from build123d import *

# Parameters (mm, degrees)
CROQUIS5_R              = 1.6
SALIENTE_EXTRUIR3_DEPTH = 15
SALIENTE_EXTRUIR5_DEPTH = 2
CORTAR_EXTRUIR3_DEPTH   = 3
CROQUIS10_W             = 4
CROQUIS10_H             = 50
SALIENTE_EXTRUIR6_DEPTH = 18
CROQUIS17_R             = 1.6
CORTAR_EXTRUIR4_DEPTH   = 4
CORTAR_EXTRUIR6_DEPTH   = 3


with BuildPart() as part:
    # Croquis5 → Saliente-Extruir3 (new body)
    with BuildSketch(Plane(origin=(0, 0, 0), x_dir=(1, 0, 0), z_dir=(0, 1, 0))):
        with BuildLine():
            Line((-65.609813571, 16.762782914), (-61.088751749, 16.762782914))
            ThreePointArc((-61.088751749, 16.762782914), (-59.34928266, 13.462782914), (-61.088751749, 10.162782914))
            Line((-61.088751749, 10.162782914), (-65.609813571, 10.162782914))
            ThreePointArc((-65.609813571, 10.162782914), (-67.34928266, 13.462782914), (-65.609813571, 16.762782914))
        make_face()
        with Locations(Location((-63.34928266, 13.462782914, 0), (0, 0, 270))):
            Circle(CROQUIS5_R, mode=Mode.SUBTRACT)
    extrude(amount=SALIENTE_EXTRUIR3_DEPTH)

    # Croquis7 → Saliente-Extruir5 (add)
    with BuildSketch(Plane(origin=(0, 15, 0), x_dir=(1, 0, 0), z_dir=(0, 1, 0))):
        Polygon((-63.34928266, 13.462782914), (-63.34928266, -11.537217086), (-71.34928266, -11.537217086), (-71.34928266, 38.462782914), (-63.34928266, 38.462782914), align=None)
    extrude(amount=-SALIENTE_EXTRUIR5_DEPTH)

    # Croquis9 → Cortar-Extruir3 (cut)
    with BuildSketch(Plane(origin=(0, 15, 0), x_dir=(1, 0, 0), z_dir=(0, 1, 0))):
        Polygon((-60.274222832, 14.551286652), (-62.754424635, 16.670114712), (-65.829484463, 15.581610975), (-66.424342488, 12.374279177), (-63.944140685, 10.255451116), (-60.869080857, 11.343954853), align=None)
    extrude(amount=-CORTAR_EXTRUIR3_DEPTH, mode=Mode.SUBTRACT)

    # Croquis10 → Saliente-Extruir6 (add)
    with BuildSketch(Plane(origin=(0, 15, 0), x_dir=(1, 0, 0), z_dir=(0, 1, 0))):
        with Locations((-69.34928266, 13.462782914)):
            Rectangle(CROQUIS10_W, CROQUIS10_H)
    extrude(amount=SALIENTE_EXTRUIR6_DEPTH)

    # Croquis17 → Cortar-Extruir4 (cut)
    with BuildSketch(Plane(origin=(-67.34928266, 0, 0), x_dir=(0, 0, -1), z_dir=(1, 0, 0))):
        with Locations((-5.037217086, 26)):
            Circle(CROQUIS17_R)
        with Locations(Location((31.962782914, 26, 0), (0, 0, 180))):
            Circle(CROQUIS17_R)
    extrude(amount=-CORTAR_EXTRUIR4_DEPTH, mode=Mode.SUBTRACT)

    # Croquis19 → Cortar-Extruir6 (cut)
    with BuildSketch(Plane.ZY.offset(71.34928266)):
        Polygon((-31.962782914, 29.233161507), (-34.762782914, 27.616580754), (-34.762782914, 24.383419246), (-31.962782914, 22.766838493), (-29.162782914, 24.383419246), (-29.162782914, 27.616580754), align=None)
        Polygon((2.237217086, 27.616580754), (5.037217086, 29.233161507), (7.837217086, 27.616580754), (7.837217086, 24.383419246), (5.037217086, 22.766838493), (2.237217086, 24.383419246), align=None)
    extrude(amount=-CORTAR_EXTRUIR6_DEPTH, mode=Mode.SUBTRACT)


solid = part.part
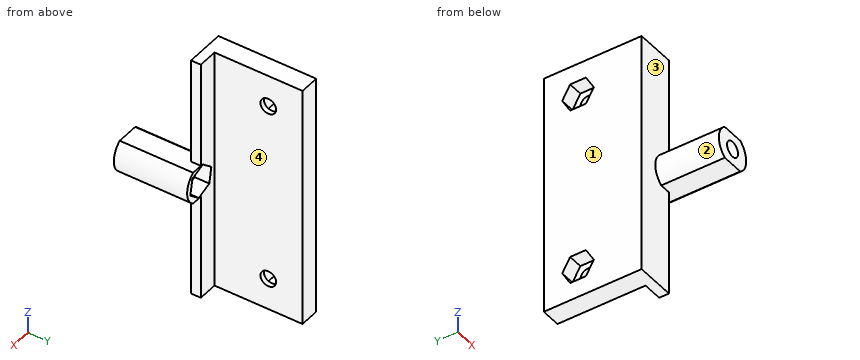
Verification items for the finished model (mm, model axes). Face numbers are marked on the shaded views. A direction names the side the tool comes from. Give positions to 0.01 mm unless a question says otherwise; leave off trailing zeros. Order: outer loops, then holes, each group sorted by start corner. A loop starts at its lowest first (then second) coordinate and runs counter-clockwise, first axis right, second up. Notation, with made-up numbers: (17.25, -17) -> (70.25, -17) arc R24 ccw to (70.25, -3) -> close; hole circle Ø4 at (-1, 78.25). An arc over 180 degrees is marked (long way). Answer as CSV lines item,"result".
Q1. Sectioned sample at C-C on z = 1.5. Record the cut outline in (x, y), plus the area to 3 significant figures.
Solutions:
outline,"(-71.35, 13) -> (-63.35, 13) -> (-63.35, 15) -> (-67.35, 15) -> (-67.35, 33) -> (-71.35, 33) -> close"
area,"88.0 mm²"
Q2. Sectioned sample at B-B on x = -69.5. Record the cut outline in (y, z), plus the area to 3 significant figures.
Solutions:
outline,"(13, -38.46) -> (33, -38.46) -> (33, 11.54) -> (13, 11.54) -> close; hole (22.77, -31.96) -> (24.38, -34.76) -> (27.62, -34.76) -> (29.23, -31.96) -> (27.62, -29.16) -> (24.38, -29.16) -> close; hole (22.77, 5.04) -> (24.38, 2.24) -> (27.62, 2.24) -> (29.23, 5.04) -> (27.62, 7.84) -> (24.38, 7.84) -> close"
area,"946 mm²"
Q3. Access from +Z, -Z, +X, -X, +Y, -Y to the whole of each face (thin tool, end or side, straight path). Record for the marked faces 1 and 2.
Solutions:
face 1,"+Z, -Z, -X, +Y, -Y"
face 2,"-X, -Y"
Q4. Depth check by flat-ended pin: pin 1 (5.5 mm diameter, centred on y = 22.5, z = -5.5, fed in from +X); pin 2 (3 mm diameter, centred on y = 25.5, z = 5.5, fed in from -X); pin 3 (6 mm diameter, centred on x = -65, y = 4.5, fed in from -Z). Enter the tip coordinate at first touch or a pass-through.
Solutions:
pin 1,"stops at x = -67.35"
pin 2,"stops at x = -68.35"
pin 3,"stops at z = -16.76"
Q5. Sectioned sample at A-A on y = 26. Record the cut outline in (x, z), plus the area to 3 significant figures.
Solutions:
outline,"(-71.35, -38.46) -> (-67.35, -38.46) -> (-67.35, -33.56) -> (-68.35, -33.56) -> (-68.35, -34.76) -> (-71.35, -34.76) -> close; (-71.35, -29.16) -> (-68.35, -29.16) -> (-68.35, -30.36) -> (-67.35, -30.36) -> (-67.35, 3.44) -> (-68.35, 3.44) -> (-68.35, 2.24) -> (-71.35, 2.24) -> close; (-71.35, 7.84) -> (-68.35, 7.84) -> (-68.35, 6.64) -> (-67.35, 6.64) -> (-67.35, 11.54) -> (-71.35, 11.54) -> close"
area,"160 mm²"
Q6. Release check for a two-part mould opening along Y. For the marked faces 3 and 4 record: +Y half, -Y half, draft (parallel to the pull), parting line (faces both ways), or undercut.
Solutions:
face 3,"-Y half"
face 4,"draft"
Q7. Scan lines: probe 1 along X at (y, z) = (20.5, -34); probe 2 along Z at (x, y) = (-61.25, 7); probe 3 along X at (y, z) = (26, -30). Record each from-to range of solid material in increasing order.
Solutions:
probe 1,"x = -71.35 to -67.35"
probe 2,"z = -16.76 to -10.16"
probe 3,"x = -68.35 to -67.35"
Q8. Sectioned sample at D-D on y = 20. Record the cut outline in (x, z), plus the area to 3 significant figures.
Solutions:
outline,"(-71.35, -38.46) -> (-67.35, -38.46) -> (-67.35, 11.54) -> (-71.35, 11.54) -> close"
area,"200 mm²"
